Could you check a few things on this model? Use its own coordinates, in mm. A direction names the side the tool comes from. Coordinates: 2 decimals unless noted, no trailing zeros. Write each loop counter-clockwise with the first axis right and the second up, starting at its lowest first coordinate (ties: lowest second). Pieces come first, ordered by that corner, then holes. Notation, with made-up numbers: M 81.5,61 L 122.5,61 A14 cw 122.5,76 Z; hole C 64.5,-11 d2. An arc over 180 degrees is marked long. Answer as CSV lines item,"result". Start each with the question number.
Item 1: Suppose I cut it at C-C, the plane y = 10. Write out the boundary of the cut face in (x, z), and give its area (3 significant figures).
Item 2: If I drill on line 1 along Y through (x, z) = (-10, 4.75); line 2 along X through (y, z) = (7, 2.15); line 3 along Z through (x, y) = (50, 16), over which ranges is the centre line in solid material (lowest first)? Write a range as [from, to].
Item 3: We'd pull the mould along Y, two halves only. Please class faces 3 (the flat face through (23, 8, 0)), 4 (the flat face through (23, 19.88, 2)), 5 (the flat face through (-24.357, 8, 3)), 6 (the flat face through (23, 18.38, 3)): +Y half, -Y half, draft (parallel to the pull), parting line (faces both ways), or undercut.
Item 4: Suppose I cut it at B-B, the plane x = 31. Write out the boundary of the cut face in (y, z), and give its area (3 significant figures).
Item 5: Suppose I cut it at A-A, the plane z = 2.85. Write out the boundary of the cut face in (x, y), and give its area (3 significant figures).
Item 6: On a 3-axis mill with a long thin cutter (end or side, diameter ignored), from which of +Z, -Z, +X, -X, +Y, -Y can I reach the whole of each face in a straight line? I mean faces 1 (the flat face through (23, -4.12, 2)), 2 (the flat face through (23, 8, 2)). Say none if no direction works.
Item 7: I'm going to push a flat-ended pin straight in: P1, Ø10, axis at x = 49, y = 11, coming from the +Z side. Where does the tip first touch, or does it pass through?
```python
from build123d import *

# Parameters (mm, degrees)
F0_W     = 100
F0_H     = 24
F0_W_2   = 97
F0_H_2   = 21
F1_DEPTH = 2
F2_DEPTH = 5
F3_R     = 1


with BuildPart() as f1:
    # F0 (on Top) → F1 (new body)
    with BuildSketch(Plane.XY):
        with Locations((24.1434355296, 7.8797731549)):
            Rectangle(F0_W, F0_H)
        with Locations((24.1434355296, 7.8797731549)):
            Rectangle(F0_W_2, F0_H_2, mode=Mode.SUBTRACT)
        with Locations((24.1434355296, 7.8797731549)):
            Rectangle(F0_W_2, F0_H_2)
    extrude(amount=F1_DEPTH)

    # F0 (on Top) → F2 (join)
    with BuildSketch(Plane.XY):
        with Locations((24.1434355296, 7.8797731549)):
            Rectangle(F0_W, F0_H)
        with Locations((24.1434355296, 7.8797731549)):
            Rectangle(F0_W_2, F0_H_2, mode=Mode.SUBTRACT)
    extrude(amount=F2_DEPTH)

    # F3
    f3_edges = [f1.edges().sort_by_distance(p)[0] for p in [
        (74.143436, 19.879773, 2.5),
        (74.143436, -4.120227, 2.5),
        (-25.856564, -4.120227, 2.5),
        (-25.856564, 19.879773, 2.5),
    ]]
    fillet(f3_edges, radius=F3_R)


solid = f1.part
```
Ans:
1,outline,"M -25.86,0 L 74.14,0 L 74.14,5 L 72.64,5 L 72.64,2 L -24.36,2 L -24.36,5 L -25.86,5 Z"
1,area,"209 mm^2"
2,line 1,"y = [-4.12, -2.62], [18.38, 19.88]"
2,line 2,"x = [-25.86, -24.36], [72.64, 74.14]"
2,line 3,"z = [0, 2]"
3,face 3,"draft"
3,face 4,"+Y half"
3,face 5,"undercut"
3,face 6,"undercut"
4,outline,"M -4.12,0 L 19.88,0 L 19.88,5 L 18.38,5 L 18.38,2 L -2.62,2 L -2.62,5 L -4.12,5 Z"
4,area,"57.0 mm^2"
5,outline,"M -25.86,-3.12 A1 ccw -24.86,-4.12 L 73.14,-4.12 A1 ccw 74.14,-3.12 L 74.14,18.88 A1 ccw 73.14,19.88 L -24.86,19.88 A1 ccw -25.86,18.88 Z; hole M -24.36,-2.62 L 72.64,-2.62 L 72.64,18.38 L -24.36,18.38 Z"
5,area,"362 mm^2"
6,face 1,"+Z, -Z, +X, -X, -Y"
6,face 2,"+Z"
7,P1,"stops at z = 2"
